Could you check a few things on this model? Use its own coordinates, in mm. Round coordinates to 2 decimals unless told otherwise and drop trailing zeros. Loops run counter-clockwise (first coordinate to the right, second up) from the corner with the lowest first, then second, coordinate; pieces in that order, holes last.
from build123d import *

# Parameters (mm, degrees)
CROQUIS1_R              = 1.5
SALIENTE_EXTRUIR1_DEPTH = 0.5


with BuildPart() as part:
    # Croquis1 → Saliente-Extruir1 (new body)
    with BuildSketch(Plane(origin=(0, 0, 0), x_dir=(1, 0, 0), z_dir=(0, 1, 0))):
        with BuildLine():
            Line((43.47, -43.46), (51.37, -43.46))
            Line((51.37, -43.46), (51.37, -51.26))
            Line((51.37, -51.26), (43.47, -51.26))
            Line((43.47, -51.26), (43.47, -67.33))
            Line((43.47, -67.33), (7.2, -97.72))
            Line((7.2, -97.72), (0, -97.72))
            ThreePointArc((0, -97.72), (-2.121320344, -96.841320344), (-3, -94.72))
            Line((-3, -94.72), (-3, 0))
            ThreePointArc((-3, 0), (-2.121320344, 2.121320344), (0, 3))
            Line((0, 3), (7.2, 3))
            Line((7.2, 3), (43.47, -27.39))
            Line((43.47, -27.39), (43.47, -43.46))
        make_face()
        with Locations(Location((0, 0, 0), (0, 0, 270))):
            Circle(CROQUIS1_R, mode=Mode.SUBTRACT)
        with Locations(Location((0, -94.72, 0), (0, 0, 270))):
            Circle(CROQUIS1_R, mode=Mode.SUBTRACT)
        with Locations(Location((47.47, -47.36, 0), (0, 0, 270))):
            Circle(CROQUIS1_R, mode=Mode.SUBTRACT)
        with Locations(Location((15.47, -23.96, 0), (0, 0, 270))):
            Circle(CROQUIS1_R, mode=Mode.SUBTRACT)
        with Locations(Location((15.47, -70.76, 0), (0, 0, 270))):
            Circle(CROQUIS1_R, mode=Mode.SUBTRACT)
    extrude(amount=SALIENTE_EXTRUIR1_DEPTH)


solid = part.part
Item 1: We'd pull the mould along X, two halves only. Please class faces 1 (the flat face through (19, 0.5, 47)), 2 (the cylindrical face through (-2.14, 0.25, -2.1)), 3 (the cylindrical face through (0.45, 0.25, 1.43)): released by +X, released by -X, zero draft, split by the parting line, or undercut.
Results list:
face 1: zero draft
face 2: released by -X
face 3: undercut
Item 2: If we section it at C-C, the plane z = 23.96: Please give me the cut outline in (x, y).
Results list:
outline: (-3, 0) - (13.97, 0) - (13.97, 0.5) - (-3, 0.5) - close; (16.97, 0) - (39.38, 0) - (39.38, 0.5) - (16.97, 0.5) - close
Item 3: If we section it at D-D, the plane x = 15.47: Please give me the cut outline in (y, z), then the cut area to 3 significant figures.
Results list:
outline: (0, 3.93) - (0.5, 3.93) - (0.5, 22.46) - (0, 22.46) - close; (0, 25.46) - (0.5, 25.46) - (0.5, 69.26) - (0, 69.26) - close; (0, 72.26) - (0.5, 72.26) - (0.5, 90.79) - (0, 90.79) - close
area: 40.4 mm2
Item 4: If we section it at B-B, the plane y = 0.4: Please give me the cut outline in (x, z), then the cut area to 3 significant figures.
Results list:
outline: (-3, 0) arc R3 ccw to (0, -3) - (7.2, -3) - (43.47, 27.39) - (43.47, 43.46) - (51.37, 43.46) - (51.37, 51.26) - (43.47, 51.26) - (43.47, 67.33) - (7.2, 97.72) - (0, 97.72) arc R3 ccw to (-3, 94.72) - close; hole circle Ø3 at (0, 0); hole circle Ø3 at (0, 94.72); hole circle Ø3 at (15.47, 23.96); hole circle Ø3 at (15.47, 70.76); hole circle Ø3 at (47.47, 47.36)
area: 3,600 mm2
Item 5: If we section it at A-A, the plane x = 47.47: Please give me the cut outline in (y, z), then the cut area to 3 significant figures.
Results list:
outline: (0, 43.46) - (0.5, 43.46) - (0.5, 45.86) - (0, 45.86) - close; (0, 48.86) - (0.5, 48.86) - (0.5, 51.26) - (0, 51.26) - close
area: 2.40 mm2
Item 6: If I drill on line 1 along X through (y, z) = (0.25, 47.36); line 2 along Z through (x, y) = (16.5, 0.4); line 3 along X through (y, z) = (0.2, 0), over which ranges is the centre line in solid material (lowest first)?
Results list:
line 1: x = -3 to 45.97, 48.97 to 51.37
line 2: z = 4.79 to 22.87, 25.05 to 69.67, 71.85 to 89.93
line 3: x = -3 to -1.5, 1.5 to 10.78
